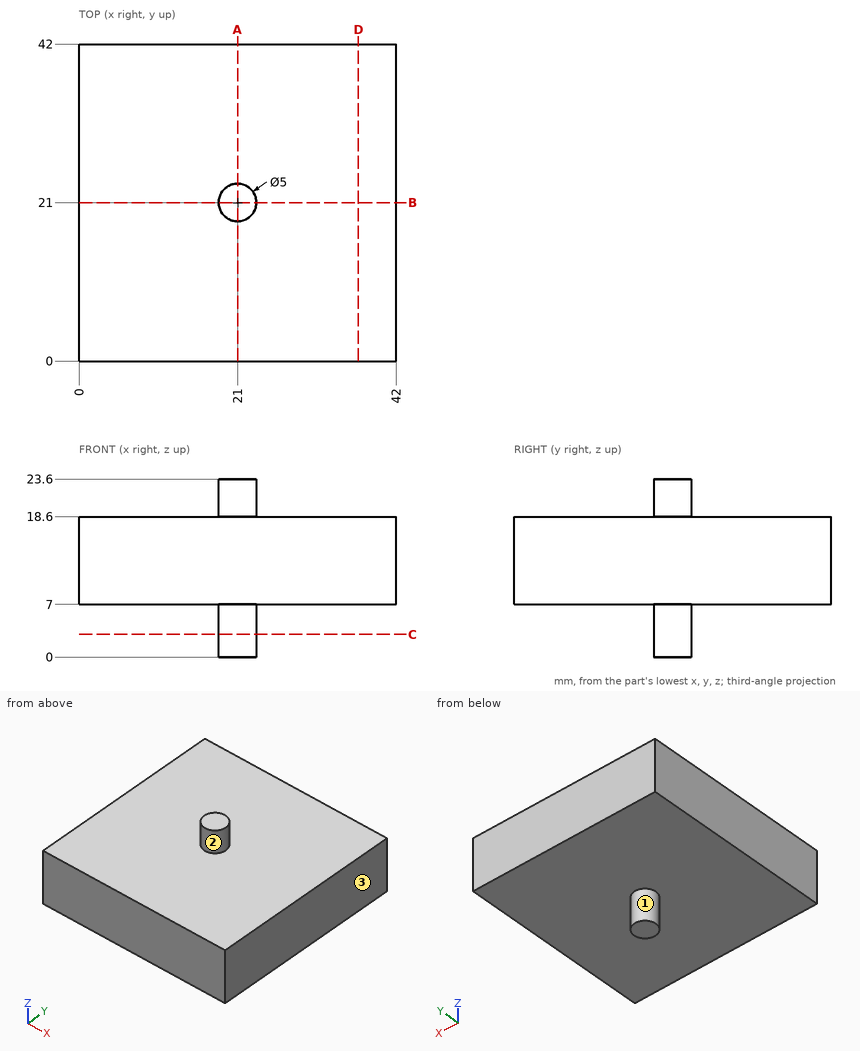
Can you work these out from the drawing? Everything is in mm from the part's minimum corner. A direction names the side the tool comes from. Give positions to 0.01 mm unless a question says otherwise; leave off trailing zeros. Loops run counter-clockwise (first coordinate to the right, second up) from the corner with the lowest first, then second, coordinate; pieces in that order, holes last. Notation, with made-up numbers: (-13, 32) -> (13, 32) arc R24 cw to (13, 57) -> close; hole circle Ø9 at (47, 19.25). An arc over 180 degrees is marked (long way). Write item = value, one per line.
1) Suppose I cut it at C-C on z = 3. Write out the boundary of the cut face in (x, y).
Check result:
outline = circle Ø5 at (21, 21)
2) Will these pins go through, and if not, where does the flat tip stop? pin 1 (1 mm diameter, centred on y = 20.5, z = 5.5, fed in from -X); pin 2 (8 mm diameter, centred on x = 22, y = 27.5, fed in from -Z); pin 3 (12 mm diameter, centred on x = 11.5, y = 21.5, fed in from +Z).
Check result:
pin_1 = 18.5
pin_2 = 7
pin_3 = 18.6
3) Suppose I cut it at D-D on x = 37. Write out the boundary of the cut face in (y, z), then the cut area to 3 significant figures.
Check result:
outline = (0, 7) -> (42, 7) -> (42, 18.6) -> (0, 18.6) -> close
area = 487 mm2
4) For the marked faces 1, 2 and 3, which set-ups out of +Z, -Z, +X, -X, +Y, -Y let a thin tool reach every point of the face, with its end or its side?
Check result:
face_1 = -Z
face_2 = +Z
face_3 = +Z, -Z, +X, +Y, -Y
5) I need wall thicknesses on L1, parallel to Z at x = 13.5, y = 13.5; L2, parallel to X at y = 21, z = 20. Which ranges of each line are inside material? Lowest first, please. Write a range as from..to.
Check result:
L1 = 7..18.6
L2 = 18.5..23.5
6) Suppose I cut it at A-A on x = 21. Write out the boundary of the cut face in (y, z).
Check result:
outline = (0, 7) -> (18.5, 7) -> (18.5, 0) -> (23.5, 0) -> (23.5, 7) -> (42, 7) -> (42, 18.6) -> (23.5, 18.6) -> (23.5, 23.6) -> (18.5, 23.6) -> (18.5, 18.6) -> (0, 18.6) -> close
